Geometry: final body of the model. Coordinates: model frame, mm. A direction names the side the tool comes from. Round coordinates to 2 decimals unless told otherwise and drop trailing zeros. Write each loop counter-clockwise with the first axis right and the second up, starting at its lowest first coordinate (ties: lowest second). Pieces come first, ordered by that corner, then holes. Notation, with made-up numbers: (-23.5, -12.5) -> (2.5, -12.5) arc R26 cw to (2.5, 9.5) -> close; hole circle Ø3 at (-14.75, 34). An arc over 180 degrees is marked (long way). One line per item, written item: value. Start each with the question number.
Autodesk Inventor part; units mm, degrees
ref_plane "YZ Plane" through (0, 0, 0) normal (1, 0, 0) x (0, 1, 0)
ref_plane "XZ Plane" through (0, 0, 0) normal (0, 1, 0) x (-1, 0, 0)
ref_plane "XY Plane" through (0, 0, 0) normal (0, 0, 1) x (1, 0, 0)
sketch "Sketch1" plane through (0, 0, 0) normal (0, 1, 0) x (-1, 0, 0)
  line L0 (20, 20) -> (20, -20)
  line L1 (20, -20) -> (-20, -20)
  line L2 (-20, -20) -> (-20, 20)
  line L3 (-20, 20) -> (20, 20)
  line L4 (-15, 15) -> (-15, -15) construction
  line L5 (-15, -15) -> (15, -15) construction
  line L6 (15, -15) -> (15, 15) construction
  line L7 (15, 15) -> (-15, 15) construction
  circle A0 centre (15, 15) radius 3.05
  circle A1 centre (15, -15) radius 3.05
  circle A2 centre (-15, -15) radius 3.05
  circle A3 centre (-15, 15) radius 3.05
  line L8 (0, 0) -> (-18.5703, 0) construction
  line L9 (0, 0) -> (0, 25.6262) construction
  line L10 (0, 0) -> (-18.05, 0) construction
  line L11 (8, 2.3333) -> (-8, 2.3333)
  line L12 (-8.5, 1.8333) -> (-8.5, 1.8333)
  line L13 (8.5, 1.8333) -> (8.5, 1.8333)
  line L14 (8.5, 2.3333) -> (-8.5, 3.0056) construction
  line L15 (-8.5, 2.3333) -> (8.5, 3.0548) construction
  arc A4 (8.5, 1.8333) -> (8, 2.3333) centre (8, 1.8333) ccw
  arc A5 (8, 1.3333) -> (8.5, 1.8333) centre (8, 1.8333) ccw
  arc A6 (-8.5, 1.8333) -> (-8, 1.3333) centre (-8, 1.8333) ccw
  arc A7 (-8, 2.3333) -> (-8.5, 1.8333) centre (-8, 1.8333) ccw
  line L16 (-8.5, -1.8333) -> (-8.5, -1.8333)
  line L17 (-8, -2.3333) -> (8, -2.3333)
  line L18 (8.5, -1.8333) -> (8.5, -1.8333)
  line L19 (8.5, -0.691) -> (-8.5, -2.3333) construction
  line L20 (-8.5, -0.6827) -> (8.5, -2.3333) construction
  arc A8 (8.5, -1.8333) -> (8.0002, -1.3333) centre (8, -1.8333) ccw
  arc A9 (8, -2.3333) -> (8.5, -1.8333) centre (8, -1.8333) ccw
  arc A10 (-8.5, -1.8333) -> (-8, -2.3333) centre (-8, -1.8333) ccw
  arc A11 (-8, -1.3333) -> (-8.5, -1.8333) centre (-8, -1.8333) ccw
  line L21 (8, 1.3333) -> (7, 1.3333)
  line L22 (7, 1.3333) -> (7, -1.3333)
  line L23 (7, -1.3333) -> (8.0002, -1.3333)
  line L24 (-8, 1.3333) -> (-7, 1.3333)
  line L25 (-7, 1.3333) -> (-7, -1.3333)
  line L26 (-7, -1.3333) -> (-8, -1.3333)
  point P0 (0, -12.01)
  point P1 (-0.3001, 2.6813)
  point P2 (0, 2.694)
  point P3 (0.0215, -1.5101)
  point P4 (0, -1.508)
  point P5 (0, -1.5122)
  dimension "d0" = 40
  dimension "d1" = 40
  dimension "d2" = 30
  dimension "d53" = 20
  dimension "d114" = 17
  dimension "d117" = 0.5
  dimension "d140" = 17
  dimension "d142" = 0.5
  dimension "d146" = 14
  dimension "d147" = 7
  dimension "d150" = 1.3333
  dimension "d151" = 1.3333
  dimension "d152" = 2.3333
  dimension "d153" = 2.3333
extrude "Extrusion15" add sketch "Sketch1" along normal blind 5
sketch "Sketch11" plane through (0, 0, 0) normal (0, -1, 0) x (1, 0, 0)
  line L0 (-11, -7.5) -> (11, -7.5)
  line L1 (12.5, -6) -> (12.5, 6)
  line L2 (11, 7.5) -> (-11, 7.5)
  line L3 (-12.5, 6) -> (-12.5, -6)
  line L4 (-12.5, -7.5) -> (12.5, 7.5) construction
  line L5 (12.5, -7.5) -> (-12.5, 7.5) construction
  arc A0 (-11, 7.5) -> (-12.5, 6) centre (-11, 6) ccw
  arc A1 (-12.5, -6) -> (-11, -7.5) centre (-11, -6) ccw
  arc A2 (11, -7.5) -> (12.5, -6) centre (11, -6) ccw
  arc A3 (12.5, 6) -> (11, 7.5) centre (11, 6) ccw
  point P0 (0, 0)
  dimension "d154" = 15
  dimension "d155" = 25
  dimension "d156" = 1.5
extrude "Extrusion16" cut sketch "Sketch11" against normal blind 3
sketch "Sketch14" plane through (0, 0, 0) normal (0, -1, 0) x (1, 0, 0)
  arc A0 (-12.5, -6) -> (-11, -7.5) centre (-11, -6) ccw
  line L0 (-12.5, -6) -> (-12.5, 6)
  arc A1 (-11, 7.5) -> (-12.5, 6) centre (-11, 6) ccw
  line L1 (-11, 7.5) -> (11, 7.5)
  arc A2 (12.5, 6) -> (11, 7.5) centre (11, 6) ccw
  line L2 (12.5, 6) -> (12.5, -6)
  arc A3 (11, -7.5) -> (12.5, -6) centre (11, -6) ccw
  line L3 (11, -7.5) -> (-11, -7.5)
  circle A4 centre (15, 15) radius 3.05
  circle A5 centre (15, -15) radius 3.05
  circle A6 centre (-15, -15) radius 3.05
  circle A7 centre (-15, 15) radius 3.05
  line L4 (-20, 20) -> (-20, -20)
  line L5 (-20, -20) -> (20, -20)
  line L6 (20, -20) -> (20, 20)
  line L7 (20, 20) -> (-20, 20)
  point P0 (0, 0)
extrude "Extrusion17" add sketch "Sketch14" along normal blind 3
sketch "Sketch12" plane through (20, 0, 20) normal (1, 0, 0) x (0, 0, -1)
  line L0 (40, 5) -> (40, -3)
  line L1 (0, 5) -> (40, 5)
  line L2 (0, 5) -> (0, -3)
  line L3 (40, -3) -> (0, -3)
  point P0 (20, 0)
  point P1 (5, 1)
  point P2 (35, 1)
  dimension "d163" = 5
  dimension "d164" = 5
  dimension "d165" = 4
  dimension "d166" = 4
hole "Hole1" at (20, 1, 15) at (20, 1, -15) direction (-1, 0, 0) diameter 2.013 depth 5 tip angle 118
sketch "Sketch13" plane through (-20, 0, -20) normal (-1, 0, 0) x (0, 0, 1)
  line L0 (40, -3) -> (40, 5)
  line L1 (0, 5) -> (40, 5)
  line L2 (0, 5) -> (0, -3)
  circle A0 centre (35, 1) radius 1.0065
  circle A1 centre (5, 1) radius 1.0065
  line L3 (40, -3) -> (0, -3)
  point P0 (20, 0)
  point P1 (33.9935, 1)
  point P2 (3.9935, 1)
hole "Hole2" at (-20, 1, 15) at (-20, 1, -15) direction (1, 0, 0) diameter 2.013 depth 5 tip angle 118
sketch "Sketch15" plane through (0, 5, 0) normal (0, 1, 0) x (1, 0, 0)
  circle A0 centre (0, -12.05) radius 3.05
  circle A1 centre (0, 12.05) radius 3.05
  point P0 (0, 0)
  dimension "d183" = 6.1
  dimension "d184" = 12.05
  dimension "d185" = 6.1
  dimension "d186" = 12.05
extrude "Extrusion18" cut sketch "Sketch15" against normal blind 10
equation "\"d1\" = d0"
properties part number "HolderStartV2"
(1) Line query: probe 1 along X at (y, z) = (2.75, -2); probe 2 along X at (y, z) = (4.75, -13.5); probe 3 along Z at (x, y) = (18.55, 1). Output: solid intervals per line, ascending.
(2) Section query A-A (z = 0). Output: boundary loops of the cut face in (x, y).
(3) Set-up query: faces 1 (the face through (-12.07, 0.04, 7.05)), 2 (the face through (18.925, 0.956, 16.006)), 3 (the face through (20, 1, 0)), 4 (the face through (7.5, 4, 1.333)). Return all of +Z, -Z, +X, -X, +Y, -Y with unobstructed straight access to the full face (end or side cutting, diameter ignored); none if empty.
(4) Section query C-C (y = 3.5). Output: boundary loops of the cut face in (x, z).
(5) Section query D-D (x = 2.5). Output: boundary loops of the cut face in (y, z).
(6) Pull-direction query (Z, two-part tool) for faces 5 (the face through (-0.3, -3, -8.6)), 6 (the face through (-15.201, 1.056, -11.957)), 7 (the face through (0, 1, -20)); classes: pulls with the +Z half, pulls with the -Z half, needs draft (parallel to the pull), parting line crosses it, or undercut.
(7) Pin query (flat end, axial travel): pin 1 (1.6 mm diameter, centred on y = 1, z = -15, fed in from -X); pin 2 (5.5 mm diameter, centred on x = 0, z = 12.05, fed in from +Y). Return the tip coordinate at first contact, or that it passes through.
(8) Section query B-B (y = 1). Count the separate pieces of the cut face and the enclosed holes in it, and give its area (3 significant figures).
Results list:
1. probe 1: x = -20 to -12.5, 12.5 to 20
1. probe 2: x = -20 to -17.66, -12.34 to -2.68, 2.68 to 12.34, 17.66 to 20
1. probe 3: z = -20 to -16.01, -13.99 to 13.99, 16.01 to 20
2. outline: (-20, -3) -> (-12.5, -3) -> (-12.5, 3) -> (-7, 3) -> (-7, 5) -> (-20, 5) -> close; (7, 3) -> (12.5, 3) -> (12.5, -3) -> (20, -3) -> (20, 5) -> (7, 5) -> close
3. face 1: -Y
3. face 2: +X
3. face 3: +Z, -Z, +X, +Y, -Y
3. face 4: +Y, -Y
4. outline: (-20, -20) -> (20, -20) -> (20, 20) -> (-20, 20) -> close; hole circle Ø6.1 at (-15, -15); hole circle Ø6.1 at (-15, 15); hole (-8, -2.33) -> (8, -2.33) arc R0.5 ccw to (8, -1.33) -> (7, -1.33) -> (7, 1.33) -> (8, 1.33) arc R0.5 ccw to (8, 2.33) -> (-8, 2.33) arc R0.5 ccw to (-8, 1.33) -> (-7, 1.33) -> (-7, -1.33) -> (-8, -1.33) arc R0.5 ccw to start; hole circle Ø6.1 at (0, -12.05); hole circle Ø6.1 at (0, 12.05); hole circle Ø6.1 at (15, -15); hole circle Ø6.1 at (15, 15)
5. outline: (-3, -20) -> (5, -20) -> (5, -13.8) -> (-3, -13.8) -> close; (-3, -10.3) -> (5, -10.3) -> (5, -2.33) -> (3, -2.33) -> (3, -7.5) -> (-3, -7.5) -> close; (-3, 7.5) -> (3, 7.5) -> (3, 2.33) -> (5, 2.33) -> (5, 10.3) -> (-3, 10.3) -> close; (-3, 13.8) -> (5, 13.8) -> (5, 20) -> (-3, 20) -> close
6. face 5: needs draft
6. face 6: undercut
6. face 7: pulls with the -Z half
7. pin 1: stops at x = -12.06
7. pin 2: passes through
8. separate pieces: 1
8. enclosed holes: 3
8. area: 1,040 mm^2
